Autodesk Inventor part; units mm, degrees
ref_plane "YZ Plane" through (0, 0, 0) normal (1, 0, 0) x (0, 1, 0)
ref_plane "XZ Plane" through (0, 0, 0) normal (0, 1, 0) x (-1, 0, 0)
ref_plane "XY Plane" through (0, 0, 0) normal (0, 0, 1) x (1, 0, 0)
sketch "Boceto1" plane through (0, 0, 0) normal (0, 1, 0) x (-1, 0, 0)
  line L0 (0, 0) -> (50, 0)
  line L1 (50, 0) -> (50, -65)
  line L2 (50, -65) -> (0, -65)
  line L3 (0, -65) -> (0, 0)
  line L4 (17.7, -45) -> (32.7, -45)
  line L5 (32.7, -45) -> (32.7, -20)
  line L6 (32.7, -20) -> (17.7, -20)
  line L7 (17.7, -20) -> (17.7, -45)
  line L8 (17.7, -45) -> (32.7, -20) construction
  line L9 (32.7, -45) -> (17.7, -20) construction
  line L10 (35.7, -17) -> (35.7, -48)
  line L11 (35.7, -48) -> (14.7, -48)
  line L12 (14.7, -48) -> (14.7, -17)
  line L13 (14.7, -17) -> (35.7, -17)
  line L14 (41, -1.5) -> (9, -1.5)
  line L15 (9, -1.5) -> (9, -14)
  line L16 (9, -14) -> (41, -14)
  line L17 (41, -14) -> (41, -1.5)
  line L18 (32.7, -32.5) -> (17.7, -32.5) construction
  line L19 (41, -7.75) -> (35.5, -7.75) construction
  line L20 (35.5, -7.75) -> (14.5, -7.75) construction
  line L21 (14.5, -7.75) -> (9, -7.75) construction
  circle A0 centre (35.5, -7.75) radius 1.4
  circle A1 centre (14.5, -7.75) radius 1.4
  line L22 (41, -63.5) -> (9, -63.5)
  line L23 (9, -63.5) -> (9, -51)
  line L24 (9, -51) -> (41, -51)
  line L25 (41, -51) -> (41, -63.5)
  circle A2 centre (35.5, -57.25) radius 1.4
  circle A3 centre (14.5, -57.25) radius 1.4
  line L26 (50, -32.5) -> (43.2, -32.5) construction
  line L27 (0, -32.5) -> (6.8, -32.5)
  line L28 (45.9347, 0) -> (45.9347, -14) construction
  line L29 (43.2, -32.5) -> (43.2, -14.5) construction
  line L30 (43.2, -14.5) -> (50, -14.5) construction
  circle A4 centre (43.2, -14.5) radius 1.4
  line L31 (25.2, -20) -> (25.2, -45) construction
  circle A5 centre (7.2, -14.5) radius 1.4
  circle A6 centre (35.5, -57.25) radius 1.4
  circle A7 centre (43.2, -50.5) radius 1.4
  circle A8 centre (7.2, -50.5) radius 1.4
  line L32 (35.5, -7.75) -> (14.5, -7.75)
  point P0 (25.2, -32.5)
  point P1 (25, -14)
  point P2 (25.2, -17)
  dimension "d0" = 65
  dimension "d1" = 50
  dimension "d2" = 25
  dimension "d3" = 15
  dimension "d4" = 3
  dimension "d5" = 12.5
  dimension "d6" = 32
  dimension "d7" = 3
  dimension "d8" = 5.5
  dimension "d9" = 5.5
  dimension "d10" = 2.8
  dimension "d11" = 2.8
  dimension "d12" = 6.8
  dimension "d13" = 6.8
  dimension "d14" = 14
  dimension "d15" = 2.8
  dimension "d30" = 36
  dimension "d31" = 36
  dimension "d32" = 1.5
extrude "Extrusión1" add sketch "Boceto1" along normal blind 3 contours L10 L11 L12 L13
extrude "Extrusión2" add sketch "Boceto1" against normal blind 4 contours L0 L1 L2 L3 | L17 L16 L15 L14 | L22 L23 L24 L25
extrude "Extrusión3" add sketch "Boceto1" along normal blind 2.25 contours L17 L16 L15 L14 | L22 L23 L24 L25
sketch "Boceto2" plane through (0, 2.25, 0) normal (0, 1, 0) x (1, 0, 0)
  line L0 (-41, 1.5) -> (-9, 1.5)
  line L1 (-25, 1.5) -> (-25, 14)
  line L2 (-9, 14) -> (-41, 14)
  line L3 (-20, 1.5) -> (-30, 1.5)
  line L4 (-30, 1.5) -> (-30, 14)
  line L5 (-30, 14) -> (-20, 14)
  line L6 (-20, 14) -> (-20, 1.5)
  line L7 (-20, 1.5) -> (-30, 14) construction
  line L8 (-30, 1.5) -> (-20, 14) construction
  line L9 (-32.7, 32.5) -> (-17.7, 32.5) construction
  line L10 (-41, 63.5) -> (-9, 63.5)
  line L11 (-9, 51) -> (-41, 51)
  line L12 (-30, 63.5) -> (-30, 51)
  line L13 (-20, 51) -> (-20, 63.5)
  point P0 (0, 0)
  point P1 (-25, 7.75)
  dimension "d22" = 10
extrude "Extrusión4" cut sketch "Boceto2" against normal blind 0.75
extrude "Extrusión5" add sketch "Boceto1" against normal blind 4 contours L7 L6 L5 L4 | L10 L11 L12 L13
sketch "Boceto3" plane through (0, 3, 0) normal (0, 1, 0) x (1, 0, 0)
  line L0 (-25.2, 20) -> (-25.2, 45) construction
  line L1 (-35.7, 17) -> (-14.7, 17)
  line L2 (-25.2, 17) -> (-25.2, 48)
  line L3 (-14.7, 48) -> (-35.7, 48)
  line L4 (-24.95, 17) -> (-25.45, 17)
  line L5 (-25.45, 17) -> (-25.45, 48)
  line L6 (-25.45, 48) -> (-24.95, 48)
  line L7 (-24.95, 48) -> (-24.95, 17)
  line L8 (-24.95, 17) -> (-25.45, 48) construction
  line L9 (-25.45, 17) -> (-24.95, 48) construction
  point P0 (0, 0)
  point P1 (-25.2, 32.5)
  point P2 (-24.95, 17)
  point P3 (-24.95, 48)
  point P4 (-25.45, 17)
  dimension "d27" = 0.5
extrude "Extrusión6" cut sketch "Boceto3" against normal blind 0.75
sketch "Boceto4" plane through (-41, 0, -1.5) normal (0, 0, 1) x (1, 0, 0)
  line L0 (16.05, 2.25) -> (15.55, 2.25)
  line L1 (21, 1.5) -> (11, 1.5)
  line L2 (-9, 0) -> (41, 0)
  line L3 (15.55, 2.25) -> (15.55, 3)
fillet "Empalme1" radius 2 4 edges at (-41, 1.125, -51) (-9, 1.125, -51) (-9, 1.125, -14) (-41, 1.125, -14)
equation "\"d9\" = d8"
equation "\"d13\" = d12"
properties part number "Molde 1FBR 0.75mm"
Source: CAD feature listing. Evaluate the final solid. Frame: model axes, mm. A direction names the side the tool comes from. Coordinates: 2 decimals unless noted, no trailing zeros. Loops run counter-clockwise (first coordinate to the right, second up) from the corner with the lowest first, then second, coordinate; pieces in that order, holes last. Notation, with made-up numbers: M 43.5,17 L 57.5,17 A24 cw 57.5,28 Z; hole C 6,18.25 d9. An arc over 180 degrees is marked long. Use a Markdown table: item, result. Add a question column.
Q1. Section query B-B, the plane z = -57.25. Return loops of the section in (x, y), and give its area (4 significant figures).
Q2. Draft query along Z for faces 4 (the flat face through (-25, -2, 0)), 5 (the cylindrical face through (-43.02, -1.97, -49.11)), 6 (the flat face through (-50, -2, -32)). Return one class per face: pulls with the +Z half, pulls with the -Z half, needs draft (parallel to the pull), parting line crosses it, or undercut.
Q3. First-contact query: pin 1 (5.5 mm diameter, centred on x = -34, z = -54.5, fed in from +Y); pin 2 (2.5 mm diameter, centred on y = 1.5, z = -8.5, fed in from +X); pin 3 (1.5 mm diameter, centred on y = 2, z = -26.5, fed in from +X). Flat tips, straight axial feed; report the tip coordinate or a pass-through.
Q4. Material intervals for L1, parallel to Z at x = -27, y = 0.5; L2, parallel to Z at x = -7.2, y = -2.55; L3, parallel to X at y = 1.25, z = -29, sorted ascending.
Q5. Section query A-A, the plane y = 0.75. Return loops of the section in (x, z), and give its area (3 significant figures).
Q6. Access query for faces 1 (the flat face through (-25, 1.5, -57)), 2 (the flat face through (-14.7, 1, -33)), 3 (the flat face through (-9, 1, -7)). Directions: +Z, -Z, +X, -X, +Y, -Y. A direction counts if a zero-diameter tool reaches every point of the face in a straight line with its end or side. Return the directions, or none.
Q7. Section query C-C, the plane x = -28. Return loops of the section in (y, z).
Q8. Section query D-D, the plane x = -7.2. Return loops of the section in (y, z), and give its area (3 significant figures).
Result:
| question | item | result |
|---|---|---|
| 1 | outline | M -50,-4 L -36.9,-4 L -36.9,2.25 L -41,2.25 L -41,0 L -50,0 Z; M -34.1,-4 L -15.9,-4 L -15.9,2.25 L -20,2.25 L -20,1.5 L -30,1.5 L -30,2.25 L -34.1,2.25 Z; M -13.1,-4 L 0,-4 L 0,0 L -9,0 L -9,2.25 L -13.1,2.25 Z |
| 1 | area | 229.5 mm2 |
| 2 | face 4 | pulls with the +Z half |
| 2 | face 5 | undercut |
| 2 | face 6 | needs draft |
| 3 | pin 1 | stops at y = 2.25 |
| 3 | pin 2 | stops at x = -9 |
| 3 | pin 3 | stops at x = -14.7 |
| 4 | L1 | z = -63.5 to -51, -48 to -45, -20 to -17, -14 to -1.5 |
| 4 | L2 | z = -65 to -51.9, -49.1 to -15.9, -13.1 to 0 |
| 4 | L3 | x = -35.7 to -32.7, -17.7 to -14.7 |
| 5 | outline | M -41,-63.5 L -9,-63.5 L -9,-53 A2 ccw -11,-51 L -39,-51 A2 ccw -41,-53 Z; M -41,-12 A2 ccw -39,-14 L -11,-14 A2 ccw -9,-12 L -9,-1.5 L -41,-1.5 Z; M -35.7,-48 L -14.7,-48 L -14.7,-17 L -35.7,-17 Z; hole C -35.5,-57.25 d2.8; hole C -35.5,-7.75 d2.8; hole M -32.7,-45 L -17.7,-45 L -17.7,-20 L -32.7,-20 Z; hole C -14.5,-57.25 d2.8; hole C -14.5,-7.75 d2.8 |
| 5 | area | 1,050 mm2 |
| 6 | face 1 | -Z, +Y |
| 6 | face 2 | +X, +Y |
| 6 | face 3 | +Z, -Z, +X, +Y |
| 7 | outline | M -4,-65 L 0,-65 L 0,-63.5 L 1.5,-63.5 L 1.5,-51 L 0,-51 L 0,-48 L 3,-48 L 3,-45 L 0,-45 L 0,-20 L 3,-20 L 3,-17 L 0,-17 L 0,-14 L 1.5,-14 L 1.5,-1.5 L 0,-1.5 L 0,0 L -4,0 Z |
| 8 | outline | M -4,-65 L 0,-65 L 0,-51.9 L -4,-51.9 Z; M -4,-49.1 L 0,-49.1 L 0,-15.9 L -4,-15.9 Z; M -4,-13.1 L 0,-13.1 L 0,0 L -4,0 Z |
| 8 | area | 238 mm2 |
